Design review of the part shown in the three views and the two pictorial views. Dimensions are in mm from the part's minimum x, y and z. Round coordinates to 2 decimals unless told otherwise and drop trailing zeros. Loops run counter-clockwise (first coordinate to the right, second up) from the corner with the lowest first, then second, coordinate; pieces in that order, holes last. Notation, with made-up numbers: M 10.25,25 L 54.25,25 A27 ccw 54.25,44 Z; hole C -12.5,41.5 d3. An arc over 180 degrees is marked long. Answer as CSV lines item,"result". Start each with the question number.
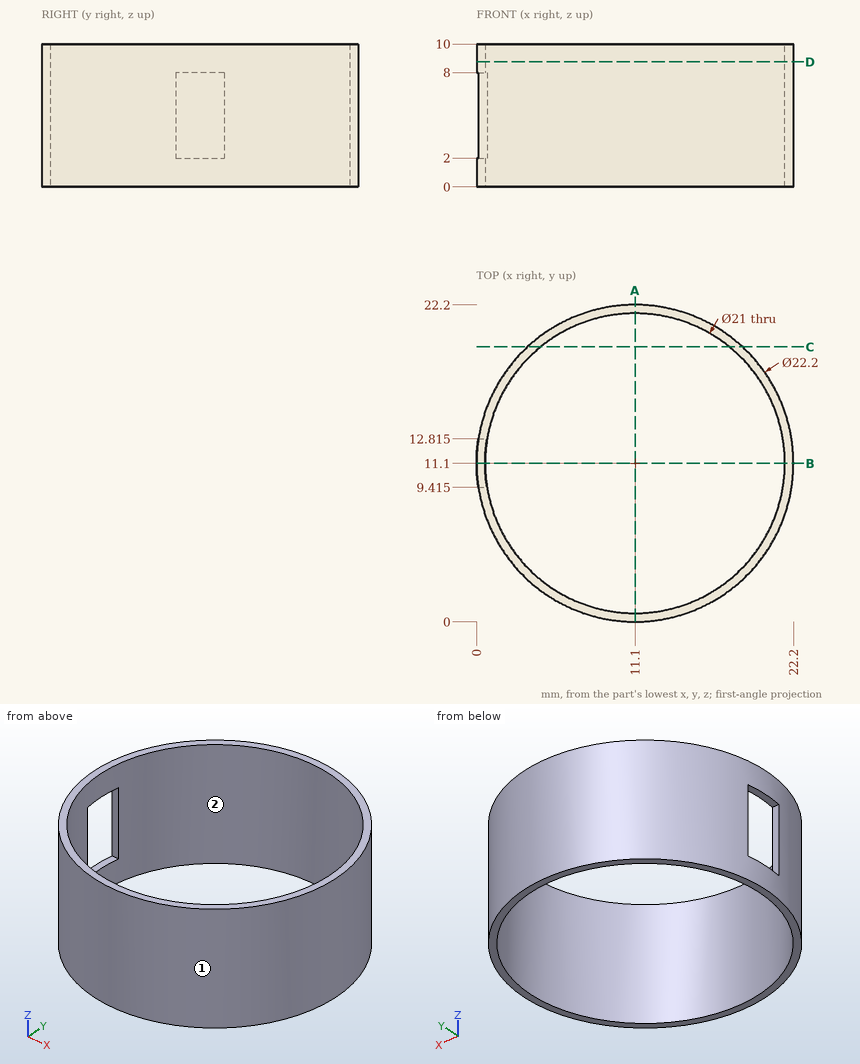
Item 1: Consider section A-A, the plane x = 11.1. Write out the cut boundary in (y, z).
Item 2: Consider section D-D, the plane z = 8.75. Write out the cut boundary in (x, y).
Item 3: Insertion check: pin 1 Ø4 at (y, z) = (4.5, 4) entering from +X; pin 2 Ø4 at (y, z) = (8, 8.5) entering from -X; pin 3 Ø5 at (y, z) = (5.5, 7) entering from -X. Each pin has a flat end and moves straight along its axis. Give the tip position at first contact, or say it passes through.
Item 4: Consider section B-B, the plane y = 11.1. Write out the cut boundary in (x, z).
Item 5: Consider section C-C, the plane y = 19.25. Write out the cut boundary in (x, z), then the cut area to 3 significant figures.
Item 6: To check wall thickness, follow line 1 (Y direction, x = 11.1, z = 7); line 2 (X direction, y = 11.1, z = 6.75). State the ranges of each line that lie inside material, in increasing order.
Item 7: The part is to be moulded in two halves that separate along X. For the marked faces 1 and 2, say which applies: +X half, -X half, draft (parallel to the pull), parting line (faces both ways), or undercut.
Found:
1,outline,"M 0,0 L 0.6,0 L 0.6,10 L 0,10 Z; M 21.6,0 L 22.2,0 L 22.2,10 L 21.6,10 Z"
2,outline,"C 11.1,11.1 d22.2; hole C 11.1,11.1 d21"
3,pin 1,"stops at x = 21.2"
3,pin 2,"stops at x = 0.05"
3,pin 3,"stops at x = 0.44"
4,outline,"M 0,0 L 0.6,0 L 0.6,2 L 0,2 Z; M 0,8 L 0.6,8 L 0.6,10 L 0,10 Z; M 21.6,0 L 22.2,0 L 22.2,10 L 21.6,10 Z"
5,outline,"M 3.56,0 L 4.48,0 L 4.48,10 L 3.56,10 Z; M 17.72,0 L 18.64,0 L 18.64,10 L 17.72,10 Z"
5,area,"18.3 mm^2"
6,line 1,"y = 0 to 0.6, 21.6 to 22.2"
6,line 2,"x = 21.6 to 22.2"
7,face 1,"parting line"
7,face 2,"undercut"
